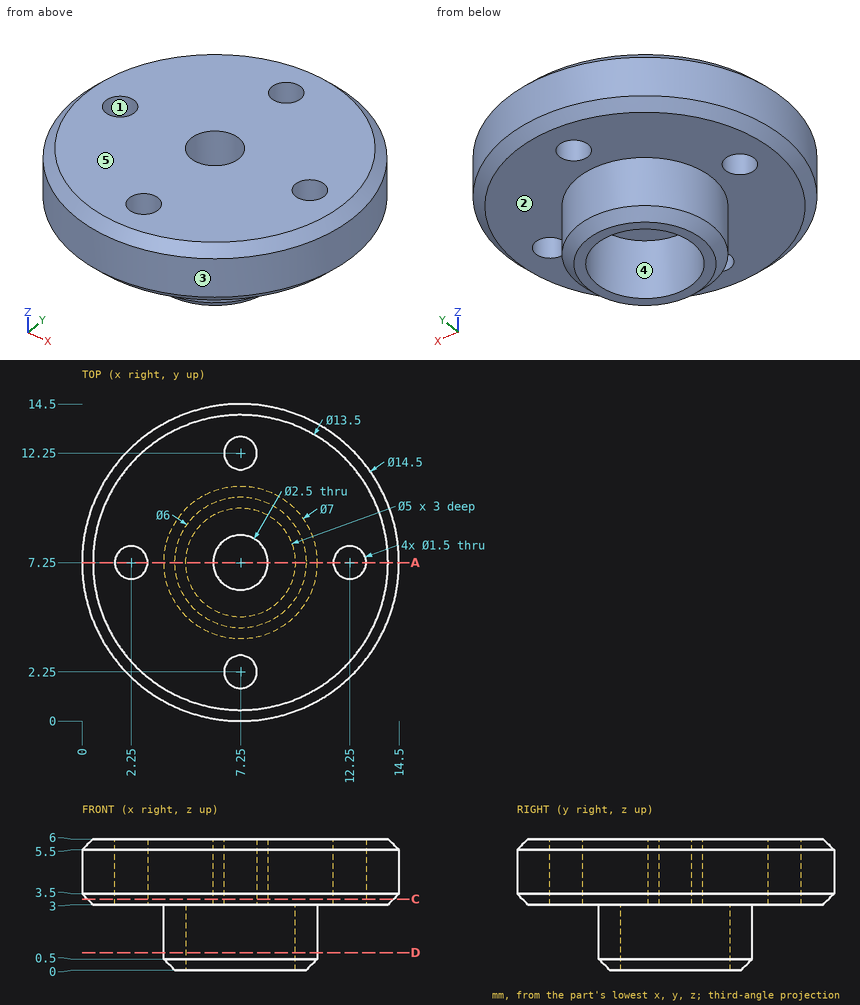
The figure shows three views and two pictorial views of one solid part (mm, origin at its lowest corner). Answer the questions. A direction names the side the tool comes from. Give positions to 0.01 mm unless a question says otherwise; leave off trailing zeros. Write each loop counter-clockwise with the first axis right and the second up, starting at its lowest first coordinate (ties: lowest second). Pieces come first, ordered by that corner, then holes. Notation, with made-up numbers: (34.25, -27) - (58.25, -27) arc R27 ccw to (58.25, -7) - close; hole circle Ø10 at (-37.5, -16). An arc over 180 degrees is marked (long way). Use one line per item in the form item = value. Start each with the question number.
1) The mould has two halves that part along X. Classify the marked faces 1, 2 and 3: pulls with the +X half, pulls with the -X half, needs draft (parallel to the pull), parting line crosses it, or undercut.
2) A tool of negligible diameter and unlimited length cuts with its end or side. For the marked faces 4 and 5, from which of +Z, -Z, +X, -X, +Y, -Y can it reach the whole face along a straight path? Write none if from no direction.
3) Find section C-C on z = 3.25. Determine the outline of the cut face in (x, y), plus the area to 3 significant figures.
4) Find section A-A on y = 7.25. Count the separate pieces of the cut face and the enclosed holes in it, plus the area to 4 significant figures.
5) Find section D-D on z = 0.8. Determine the outline of the cut face in (x, y), plus the area to 3 significant figures.
6) Flat-ended cylindrical pins translate along their axes: pin 1 Ø1 at (x, z) = (9.5, 3) entering from -Y; pin 2 Ø3 at (x, y) = (7.25, 7.25) entering from -Z; pin 3 Ø3 at (x, z) = (2, 4.5) entering from -Y. Find the tip coordinate at first contact, or state that the pin passes through.
7) Consider line 1 along Y through (x, z) = (7.25, 5.15); line 2 along Y through (x, z) = (7.25, 1.8); line 3 along Z through (x, y) = (3.5, 7.5). Determine where each line is inside the solid, lowest interval first. Write a range as from..to.
Geometry results:
q1.face_1 = undercut
q1.face_2 = needs draft
q1.face_3 = parting line crosses it
q2.face_4 = -Z
q2.face_5 = +Z, +X, -X, +Y, -Y
q3.outline = circle Ø14 at (7.25, 7.25); hole circle Ø1.5 at (2.25, 7.25); hole circle Ø2.5 at (7.25, 7.25); hole circle Ø1.5 at (7.25, 2.25); hole circle Ø1.5 at (7.25, 12.25); hole circle Ø1.5 at (12.25, 7.25)
q3.area = 142 mm2
q4.separate_pieces = 4
q4.enclosed_holes = 0
q4.area = 32.25 mm2
q5.outline = circle Ø7 at (7.25, 7.25); hole circle Ø5 at (7.25, 7.25)
q5.area = 18.8 mm2
q6.pin_1 = 0.33
q6.pin_2 = 3
q6.pin_3 = 1.05
q7.line_1 = 0..1.5, 3..6, 8.5..11.5, 13..14.5
q7.line_2 = 3.75..4.75, 9.75..10.75
q7.line_3 = 3..6
